Input: part model. Units: mm. Frame: model coordinates. A direction names the side the tool comes from. Give positions to 0.01 mm unless a question says otherwise; leave off trailing zeros. Loops run counter-clockwise (first coordinate to the right, second up) from the corner with the lowest first, then second, coordinate; pieces in that order, holes last.
from build123d import *

# Parameters (mm, degrees)
SKETCH_W     = 100
SKETCH_H     = 8
PAD_DEPTH    = 0.5
PAD001_DEPTH = 5


with BuildPart() as part:
    # Sketch → Pad (new body)
    with BuildSketch(Plane.XY):
        with Locations((50, 4)):
            Rectangle(SKETCH_W, SKETCH_H)
    extrude(amount=PAD_DEPTH)

    # Sketch001 (on Face6 of Pad) → Pad001 (join)
    with BuildSketch(Plane.XY.offset(0.5)):
        Polygon((5, 4.2), (5, 3.8), (15, 3.8), (15, 3.75), (25, 3.75), (25, 3.7), (35, 3.7), (35, 3.65), (45, 3.65), (45, 3.6), (55, 3.6), (55, 3.55), (65, 3.55), (65, 3.5), (75, 3.5), (75, 3.45), (85, 3.45), (85, 3.4), (95, 3.4), (95, 4.6), (85, 4.6), (85, 4.55), (75, 4.55), (75, 4.5), (65, 4.5), (65, 4.45), (55, 4.45), (55, 4.4), (45, 4.4), (45, 4.35), (35, 4.35), (35, 4.3), (25, 4.3), (25, 4.25), (15, 4.25), (15, 4.2), align=None)
    extrude(amount=PAD001_DEPTH)


solid = part.part
(1) Cut plane B-B (x = 60). Return the cut outline in (y, z), and give its area (3 significant figures).
Values follow:
outline: (0, 0) - (8, 0) - (8, 0.5) - (4.45, 0.5) - (4.45, 5.5) - (3.55, 5.5) - (3.55, 0.5) - (0, 0.5) - close
area: 8.50 mm2
(2) Cut plane C-C (y = 2.5). Return the cut outline in (x, z).
Values follow:
outline: (0, 0) - (100, 0) - (100, 0.5) - (0, 0.5) - close
(3) Pin query (flat end, axial travel): pin 1 Ø3 at (x, y) = (15.5, 2) entering from -Z; pin 2 Ø2.5 at (x, z) = (77.5, 3.5) entering from -Y; pin 3 Ø2.5 at (x, z) = (30, 2.5) entering from -Y; pin 4 Ø1 at (x, y) = (38.5, 2.5) entering from +Z. Return the tip coordinate at first contact, or that it passes through.
Values follow:
pin 1: stops at z = 0
pin 2: stops at y = 3.45
pin 3: stops at y = 3.7
pin 4: stops at z = 0.5
(4) Cut plane A-A (x = 28). Return the cut outline in (y, z), and give its area (3 significant figures).
Values follow:
outline: (0, 0) - (8, 0) - (8, 0.5) - (4.3, 0.5) - (4.3, 5.5) - (3.7, 5.5) - (3.7, 0.5) - (0, 0.5) - close
area: 7.00 mm2
(5) Ray query, probe 1 along Z at (x, y) = (66, 5.5); probe 2 along Y at (x, z) = (33, 3.5); probe 3 along Y at (x, z) = (21.5, 2.95). Return the intervals inside material, ascending.
Values follow:
probe 1: z = 0 to 0.5
probe 2: y = 3.7 to 4.3
probe 3: y = 3.75 to 4.25
(6) Reachability of faces 1 (the flat face through (30, 4.3, 3)), 2 (the flat face through (90, 4.6, 3)), 3 (the flat face through (70, 3.5, 3)), 4 (the flat face through (90, 3.4, 3)) from +Z, -Z, +X, -X, +Y, -Y: full face, straight path, thin tool, end or side. Return the list, or none.
Values follow:
face 1: +Z, -X, +Y
face 2: +Z, +X, -X, +Y
face 3: +Z, -X, -Y
face 4: +Z, +X, -X, -Y
